Check sheet for the modelled part. Datum: model origin and axes. Units: mm. Round coordinates to 2 decimals unless told otherwise and drop trailing zeros. Loops run counter-clockwise (first coordinate to the right, second up) from the corner with the lowest first, then second, coordinate; pieces in that order, holes last. Notation, with made-up numbers: (3.5, 36) -> (52.5, 36) arc R20 cw to (52.5, 41) -> close; hole circle Ø9 at (89.5, 5.5). An arc over 180 degrees is marked (long way). One line per item, written item: value. Start each with the question number.
1. Cross-section at C-C on x = 95.25. Record the cut outline in (y, z).
2. Cross-section at D-D on z = 15.75. Record the cut outline in (x, y) (3 decimals), then the cut area to 3 significant figures.
3. Release check for a two-part mould opening along X. For faces 1 (the face through (107.643, -70.827, 9.392)), 2 (the face through (2, -115, 0)), 3 (the face through (1.7, -146.9, 9.4)) record: +X half, -X half, draft (parallel to the pull), parting line (faces both ways), or undercut.
4. Go/stop test with flat-tipped pins: pin 1 (3 mm diameter, centred on x = 32, z = 2, fed in from -Y); pin 2 (6 mm diameter, centred on y = -108.5, z = 7, fed in from -X); pin 3 (6 mm diameter, centred on y = -129.5, z = 6, fed in from +X); pin 4 (8 mm diameter, centred on x = 89.5, y = -106, fed in from -Z). Record where each tip stops, or that it passes through.
5. Cross-section at A-A on y = -83. Record the cut outline in (x, z).
6. Material ranges on L1, parallel to X at y = -77, z = 8; L2, parallel to X at y = -84.5, z = 17; L3, parallel to Y at x = 95.25, z = 15.25, recorded low to high.
7. Cross-section at B-B on y = -101. Record the cut outline in (x, z).
from build123d import *

# Parameters (mm, degrees)
SKETCH1_R           = 9.525
BOSS_EXTRUDE1_DEPTH = 19.05


with BuildPart() as part:
    # Sketch1 → Boss-Extrude1 (new body)
    with BuildSketch(Plane.XY):
        with BuildLine():
            ThreePointArc((81.058378375, -72.585965178), (107.958279807, -71.10262336), (109.441621625, -98.002524792))
            ThreePointArc((109.441621625, -98.002524792), (0, -146.908010025), (-109.441621625, -98.002524792))
            ThreePointArc((-109.441621625, -98.002524792), (-107.958279807, -71.10262336), (-81.058378375, -72.585965178))
            ThreePointArc((-81.058378375, -72.585965178), (0, -108.808010025), (81.058378375, -72.585965178))
        make_face()
        with Locations(Location((-95.25, -85.294244985, 0), (0, 0, 180))):
            Circle(SKETCH1_R, mode=Mode.SUBTRACT)
        with Locations(Location((95.25, -85.294244985, 0), (0, 0, 180))):
            Circle(SKETCH1_R, mode=Mode.SUBTRACT)
    extrude(amount=BOSS_EXTRUDE1_DEPTH)


solid = part.part
Taken from the geometry:
1. outline: (-111.85, 0) -> (-94.82, 0) -> (-94.82, 19.05) -> (-111.85, 19.05) -> close; (-75.77, 0) -> (-66.24, 0) -> (-66.24, 19.05) -> (-75.77, 19.05) -> close
2. outline: (-109.442, -98.003) arc R146.908 ccw to (109.442, -98.003) arc R19.05 ccw to (81.058, -72.586) arc R108.808 cw to (-81.058, -72.586) arc R19.05 ccw to start; hole circle Ø19.05 at (-95.25, -85.294); hole circle Ø19.05 at (95.25, -85.294)
2. area: 8,760 mm2
3. face 1: undercut
3. face 2: draft
3. face 3: parting line
4. pin 1: stops at y = -143.71
4. pin 2: stops at x = -102.23
4. pin 3: stops at x = 74.7
4. pin 4: stops at z = 0
5. outline: (-114.16, 0) -> (-104.49, 0) -> (-104.49, 19.05) -> (-114.16, 19.05) -> close; (-86.01, 0) -> (-70.36, 0) -> (-70.36, 19.05) -> (-86.01, 19.05) -> close; (70.36, 0) -> (86.01, 0) -> (86.01, 19.05) -> (70.36, 19.05) -> close; (104.49, 0) -> (114.16, 0) -> (114.16, 19.05) -> (104.49, 19.05) -> close
6. L1: x = -112.4 to -99.93, -90.57 to -76.88, 76.88 to 90.57, 99.93 to 112.4
6. L2: x = -114.28 to -104.74, -85.76 to -68.55, 68.55 to 85.76, 104.74 to 114.28
6. L3: y = -111.85 to -94.82, -75.77 to -66.24
7. outline: (-106.68, 0) -> (-40.47, 0) -> (-40.47, 19.05) -> (-106.68, 19.05) -> close; (40.47, 0) -> (106.68, 0) -> (106.68, 19.05) -> (40.47, 19.05) -> close
